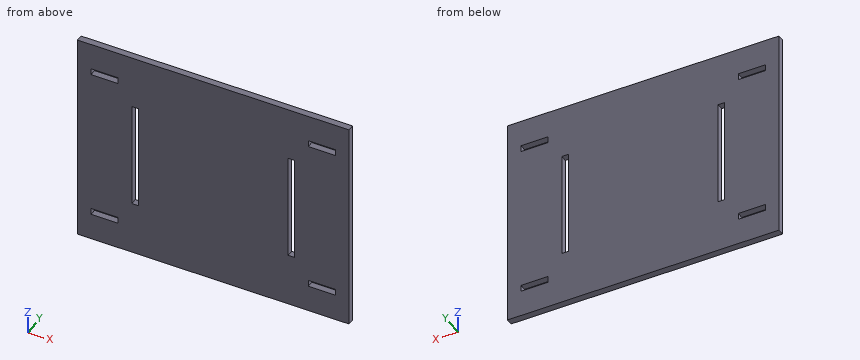
from build123d import *

# Parameters (mm, degrees)
SKETCH1_W                                  = 500
SKETCH1_H                                  = 400
BOSS_EXTRUDE1_DEPTH                        = 12
SKETCH2_W                                  = 12
SKETCH2_H                                  = 200
CUT_EXTRUDE1_DEPTH                         = 12
SKETCH5_W                                  = 50
SKETCH5_H                                  = 12
CUT_EXTRUDE2_DEPTH                         = 12
MIRROR5_AT_THE_SECOND_PLANE_COPY_1_SKETC_W = 50
MIRROR5_AT_THE_SECOND_PLANE_COPY_1_SKETC_H = 12
MIRROR5_AT_THE_SECOND_PLANE_COPY_1_DEPTH   = 12


with BuildPart() as part:
    # Sketch1 → Boss-Extrude1 (new body)
    with BuildSketch(Plane(origin=(0, 0, 0), x_dir=(1, 0, 0), z_dir=(0, 1, 0))):
        Rectangle(SKETCH1_W, SKETCH1_H)
    extrude(amount=BOSS_EXTRUDE1_DEPTH)

    # Sketch2 → Cut-Extrude1 (cut)
    with BuildSketch(Plane(origin=(0, 12, 0), x_dir=(1, 0, 0), z_dir=(0, 1, 0))):
        with Locations((-144, 0)):
            Rectangle(SKETCH2_W, SKETCH2_H)
    cut_extrude1 = extrude(amount=-CUT_EXTRUDE1_DEPTH, mode=Mode.SUBTRACT)

    # Mirror2: Cut-Extrude1 across plane
    add(cut_extrude1.mirror(Plane(origin=(0, 0, 0), x_dir=(0, 0, 1), z_dir=(1, 0, 0))), mode=Mode.SUBTRACT)

    # Sketch5 → Cut-Extrude2 (cut)
    with BuildSketch(Plane(origin=(0, 12, 0), x_dir=(1, 0, 0), z_dir=(0, 1, 0))):
        with Locations((-200, 144)):
            Rectangle(SKETCH5_W, SKETCH5_H)
    cut_extrude2 = extrude(amount=-CUT_EXTRUDE2_DEPTH, mode=Mode.SUBTRACT)

    # Mirror5: Cut-Extrude2 across plane
    add(cut_extrude2.mirror(Plane.XY), mode=Mode.SUBTRACT)

    # Mirror5 at the second plane: Cut-Extrude2 across plane
    add(cut_extrude2.mirror(Plane(origin=(0, 0, 0), x_dir=(0, 0, 1), z_dir=(1, 0, 0))), mode=Mode.SUBTRACT)

    # Mirror5 at the second plane copy 1 sketc → Mirror5 at the second plane copy 1 (cut)
    with BuildSketch(Plane(origin=(0, 12, 0), x_dir=(-1, 0, 0), z_dir=(0, 1, 0))):
        with Locations((-200, 144)):
            Rectangle(MIRROR5_AT_THE_SECOND_PLANE_COPY_1_SKETC_W, MIRROR5_AT_THE_SECOND_PLANE_COPY_1_SKETC_H)
    extrude(amount=-MIRROR5_AT_THE_SECOND_PLANE_COPY_1_DEPTH, mode=Mode.SUBTRACT)


solid = part.part
The listing builds one solid part. Answer for the finished solid, in the listing's coordinates (mm). Coordinates: 2 decimals unless noted, no trailing zeros. Write each loop counter-clockwise with the first axis right and the second up, starting at its lowest first coordinate (ties: lowest second). Pieces come first, ordered by that corner, then holes. Notation, with made-up numbers: (85, 61) - (131, 61) arc R31 ccw to (131, 94) - close; hole circle Ø6 at (55, 44). An arc over 180 degrees is marked (long way). Put each result on its own line as item: value.
1. Find the intervals of material crossed by line 1 along X through (y, z) = (1, 78.5); line 2 along X through (y, z) = (1, -144); line 3 along Z through (x, y) = (-185.5, 2.75), in increasing order. Write a range as from..to.
Answer sheet:
line 1: x = -250..-150, -138..138, 150..250
line 2: x = -250..-225, -175..175, 225..250
line 3: z = -200..-150, -138..138, 150..200
2. The part is cut by section D-D on x = 218. Give the vertices of the cut face in (y, z), plus the area to 3 significant figures.
Answer sheet:
outline: (0, -200) - (12, -200) - (12, -150) - (0, -150) - close; (0, -138) - (12, -138) - (12, 138) - (0, 138) - close; (0, 150) - (12, 150) - (12, 200) - (0, 200) - close
area: 4,510 mm^2
3. The part is cut by section A-A on x = 144.5. Give the vertices of the cut face in (y, z).
Answer sheet:
outline: (0, -200) - (12, -200) - (12, -100) - (0, -100) - close; (0, 100) - (12, 100) - (12, 200) - (0, 200) - close
4. The part is cut by section B-B on z = -44.5. Give the vertices of the cut face in (x, y), plus the area to 3 significant figures.
Answer sheet:
outline: (-250, 0) - (-150, 0) - (-150, 12) - (-250, 12) - close; (-138, 0) - (138, 0) - (138, 12) - (-138, 12) - close; (150, 0) - (250, 0) - (250, 12) - (150, 12) - close
area: 5,710 mm^2
5. The part is cut by section C-C on y = 10. Give the vertices of the cut face in (x, z), plus the area to 3 significant figures.
Answer sheet:
outline: (-250, -200) - (250, -200) - (250, 200) - (-250, 200) - close; hole (-225, -150) - (-175, -150) - (-175, -138) - (-225, -138) - close; hole (-225, 138) - (-175, 138) - (-175, 150) - (-225, 150) - close; hole (-150, -100) - (-138, -100) - (-138, 100) - (-150, 100) - close; hole (138, -100) - (150, -100) - (150, 100) - (138, 100) - close; hole (175, -150) - (225, -150) - (225, -138) - (175, -138) - close; hole (175, 138) - (225, 138) - (225, 150) - (175, 150) - close
area: 193,000 mm^2
